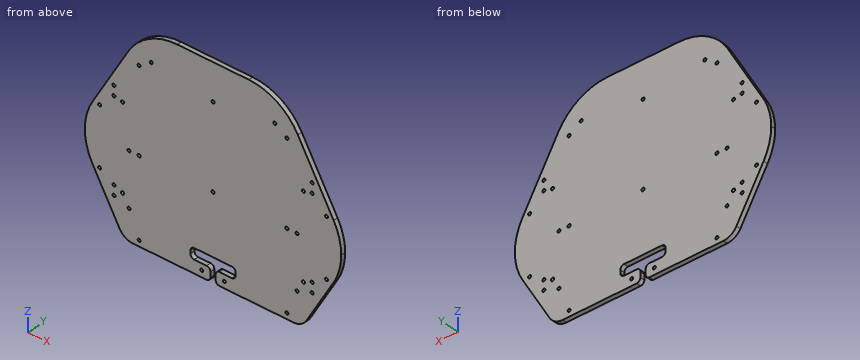
```python
from build123d import *

# Parameters (mm, degrees)
BOSS_EXTRUDE1_DEPTH    = 6
CUT_EXTRUDE1_DEPTH     = 232.669185723
M3_5_CLEARANCE_HOLE1_D = 4.199808185
M3_5_CLEARANCE_HOLE2_D = 3.949622561
FILLET1_R              = 5.024738629
FILLET2_R              = 19.924521471
FILLET3_R              = 74.958538247


with BuildPart() as part:
    # Sketch1 → Boss-Extrude1 (new body)
    with BuildSketch(Plane(origin=(0, 6, 0), x_dir=(1, 0, 0), z_dir=(0, 1, 0))):
        with BuildLine():
            Line((118.094019457, 109.999994984), (-118.094002078, 109.999994984))
            Line((-118.094002078, 109.999994984), (-159.951896595, 37.499994984))
            add(Edge.make_bspline(
                [(-159.951896595, 37.499994984), (-162.089834317, 33.796773054), (-165.842582605, 25.786056062), (-169.244504237, 13.08991169), (-169.999887381, 4.276053128), (-169.999989967, 0)],
                knots=[5.759586536, 5.759586536, 5.759586536, 5.759586536, 5.930628798, 6.11214304, 6.283185303, 6.283185303, 6.283185303, 6.283185303], degree=3))
            add(Edge.make_bspline(
                [(-169.999989967, 0), (-169.999887381, -4.276053128), (-169.244504237, -13.089911689), (-165.842582605, -25.786056062), (-162.089834317, -33.796773054), (-159.951896595, -37.499994984)],
                knots=[4e-09, 4e-09, 4e-09, 4e-09, 0.171042267, 0.352556509, 0.523598771, 0.523598771, 0.523598771, 0.523598771], degree=3))
            Line((-159.951896595, -37.499994984), (-90.801270189, -157.27241336))
            Line((-90.801270189, -157.27241336), (90.801270189, -157.27241336))
            Line((90.801270189, -157.27241336), (159.951905284, -37.5))
            add(Edge.make_bspline(
                [(159.951905284, -37.5), (162.089843006, -33.79677807), (165.842591294, -25.786061079), (169.244512926, -13.089916706), (169.99989607, -4.276058145), (169.999998656, -5.016e-06)],
                knots=[2.617993882, 2.617993882, 2.617993882, 2.617993882, 2.789036145, 2.970550387, 3.141592649, 3.141592649, 3.141592649, 3.141592649], degree=3))
            add(Edge.make_bspline(
                [(169.999998656, -5.016e-06), (169.99989607, 4.276048112), (169.244512926, 13.089906673), (165.842591294, 25.786051046), (162.089843006, 33.796768038), (159.951905284, 37.499989968)],
                knots=[3.141592658, 3.141592658, 3.141592658, 3.141592658, 3.31263492, 3.494149162, 3.665191425, 3.665191425, 3.665191425, 3.665191425], degree=3))
            Line((159.951905284, 37.499989968), (118.094019457, 109.999994984))
        make_face()
    extrude(amount=-BOSS_EXTRUDE1_DEPTH)

    # Sketch2 → Cut-Extrude1 (cut, through all)
    with BuildSketch(Plane.XZ):
        Polygon((3.5, -110), (3.5, -93), (30, -93), (30, -79), (-30, -79), (-30, -93), (-3.5, -93), (-3.5, -110), align=None)
    extrude(amount=-CUT_EXTRUDE1_DEPTH, mode=Mode.SUBTRACT)

    # M3.5 Clearance Hole1 (through all)
    with Locations(Plane(origin=(0, 0, 0), x_dir=(-1, 0, 0), z_dir=(0, -1, 0))):
        with Locations((0, -0.001547229), (-97.9932, 0.001547229), (97.9932, 0.001547229), (120, 55.001547229), (-120, 55.001547229)):
            Hole(M3_5_CLEARANCE_HOLE1_D / 2)

    # M3.5 Clearance Hole2 (through all)
    with Locations(Plane(origin=(0, 0, 0), x_dir=(-1, 0, 0), z_dir=(0, -1, 0))):
        with Locations((98, 102.43824134), (0, -109.21995866), (98, -109.21995866), (-98, -109.21995866), (111.4552, 69.84995866), (111.4552, -4.134e-05), (-111.4552, 69.84995866), (-111.4552, -4.134e-05), (-120, -55.00004134), (120, -55.00004134), (131.4, 50.30004134), (-131.4, 50.30004134), (131.4, -70.19995866), (-131.4, -70.19995866), (131.4, 63.00004134), (-131.4, 63.00004134), (131.4, -57.49995866), (-131.4, -57.49995866), (15, 101.50004134), (-98, 102.43824134), (-15, 101.50004134), (150.47, 38.10004134), (150.47, -38.09995866), (-150.47, 38.10004134), (-150.47, -38.09995866), (-82, -119.99995866), (82, -119.99995866)):
            Hole(M3_5_CLEARANCE_HOLE2_D / 2)

    # Fillet1
    fillet1_edges = [part.edges().sort_by_distance(p)[0] for p in [
        (-3.5, 3, -109.999994984),
        (-30, 3, -79),
        (30, 3, -79),
        (3.5, 3, -109.999994984),
        (-30, 3, -93),
        (-3.5, 3, -93),
        (30, 3, -93),
        (3.5, 3, -93),
    ]]
    fillet(fillet1_edges, radius=FILLET1_R)

    # Fillet2
    fillet2_edges = [part.edges().sort_by_distance(p)[0] for p in [
        (118.094019457, 3, -109.999994984),
        (-118.094002078, 3, -109.999994984),
    ]]
    fillet(fillet2_edges, radius=FILLET2_R)

    # Fillet3
    fillet3_edges = [part.edges().sort_by_distance(p)[0] for p in [
        (90.801270189, 3, 157.27241336),
        (-90.801270189, 3, 157.27241336),
    ]]
    fillet(fillet3_edges, radius=FILLET3_R)


solid = part.part
```
The model under review builds one solid part; all positions refer to its coordinate system, in mm. Round coordinates to 2 decimals unless told otherwise and drop trailing zeros. Order: outer loops, then holes, each group sorted by start corner. A loop starts at its lowest first (then second) coordinate and runs counter-clockwise, first axis right, second up.
(1) Take a section at C-C, the plane z = 138. State the section outline as (x, y) points.
Working result:
outline: (-97.7, 0) - (97.7, 0) - (97.7, 6) - (-97.7, 6) - close
(2) Take a section at B-B, the plane y = 4. Count the separate pieces of the cut face and the enclosed holes in it, plus the area to 3 significant figures.
Working result:
separate pieces: 1
enclosed holes: 32
area: 73,200 mm2
(3) For P1, Ø1, axis at y = 3.5, z = -69.5, coming from the -X side; P2, Ø4.5, axis at x = 131.4, z = 57.5, coming from the +Y side; P3, Ø3, axis at x = 131.4, z = 70.2, coming from the +Y side; P4, Ø1.5, axis at y = 1, z = -55, coming from the +X side, all flat-tipped, find the tip position at first contact; note any pin that passes through.
Working result:
P1: stops at x = -141.77
P2: stops at y = 6
P3: passes through
P4: stops at x = 150.28
(4) Take a section at A-A, the plane x = 21. State the section outline as (y, z) points.
Working result:
outline: (0, -110) - (6, -110) - (6, -93) - (0, -93) - close; (0, -79) - (6, -79) - (6, 157.27) - (0, 157.27) - close
(5) Wall thickness on L1, parallel to Z at x = -15, y = 2.2; L2, parallel to Z at x = -98, y = 1.5; L3, parallel to Z at x = -13.5, y = 3.75: over which ranges is each line inside the solid? List them lowest first.
Working result:
L1: z = -110 to -103.47, -99.53 to -93, -79 to 157.27
L2: z = -110 to -104.41, -100.46 to -2.1, 2.1 to 107.25, 111.19 to 137.73
L3: z = -110 to -102.78, -100.22 to -93, -79 to 157.27
